The listing builds one solid part. Answer for the finished solid, in the listing's coordinates (mm). A direction names the side the tool comes from. Coordinates: 2 decimals unless noted, no trailing zeros. Order: outer loops, then holes, each group sorted by start corner. A loop starts at its lowest first (then second) coordinate and runs counter-clockwise, first axis right, second up.
from build123d import *

# Parameters (mm, degrees)
SALIENTE_EXTRUIR1_DEPTH = 8
REDONDEO3_R             = 5
REDONDEO4_R             = 5
REDONDEO5_R             = 35
REDONDEO6_R             = 10
REDONDEO7_R             = 10
VACIADO1_T              = -2
CROQUIS2_R              = 2
SALIENTE_EXTRUIR2_DEPTH = 6
CROQUIS3_R              = 5
CORTAR_EXTRUIR1_DEPTH   = 10
CROQUIS4_R              = 2
SALIENTE_EXTRUIR4_DEPTH = 6
CORTAR_EXTRUIR2_START   = 10
CORTAR_EXTRUIR2_DEPTH   = 10
CROQUIS6_R              = 2
SALIENTE_EXTRUIR5_DEPTH = 6
CROQUIS7_R              = 2.5
CORTAR_EXTRUIR3_DEPTH   = 10
CORTAR_EXTRUIR4_DEPTH   = 5
REDONDEO8_R             = 2


with BuildPart() as part:
    # Croquis1 → Saliente-Extruir1 (new body)
    with BuildSketch(Plane(origin=(0, 0, 0), x_dir=(1, 0, 0), z_dir=(0, 1, 0))):
        Polygon((-30, 0), (-30, 6.559995295), (-20.5612792, 13.970160587), (0, 5.719083833), (20.5612792, 13.970160587), (30, 6.559995295), (30, 0), (0, -34.662162162), align=None)
    extrude(amount=SALIENTE_EXTRUIR1_DEPTH)

    # Redondeo3
    redondeo3_edges = [part.edges().sort_by_distance(p)[0] for p in [
        (0, 4, 34.662162162),
    ]]
    fillet(redondeo3_edges, radius=REDONDEO3_R)

    # Redondeo4
    redondeo4_edges = [part.edges().sort_by_distance(p)[0] for p in [
        (-20.5612792, 4, -13.970160587),
        (20.5612792, 4, -13.970160587),
    ]]
    fillet(redondeo4_edges, radius=REDONDEO4_R)

    # Redondeo5
    # the kernel refuses this fillet: 35 mm, written as the material it takes off along each edge
    with BuildSketch(Plane(origin=(-30, -29.587762227, 0), x_dir=(0.6544253650435297, 0, 0.7561266042056997), z_dir=(0, 1, 0))) as redondeo5_piece_1:
        with BuildLine():
            CenterArc((11.835104891, 35), REDONDEO5_R, 241.323383223, 28.676616777)
            Line((-4.960186966, 4.293027316), (-5.296092803, 3.678887862))
            ThreePointArc((-5.296092803, 3.678887862), (-2.938191238, 1.617225035), (-0.458097756, -0.529288623))
            Line((-0.458097756, -0.529288623), (0, -0.7))
            Line((0, -0.7), (11.835104891, -0.7))
            Line((11.835104891, -0.7), (11.835104891, 0))
        make_face()
    extrude(amount=67.175524454, mode=Mode.SUBTRACT)
    with BuildSketch(Plane(origin=(30, -29.587762227, 0), x_dir=(0, 0, -1), z_dir=(0, 1, 0))) as redondeo5_piece_2:
        with BuildLine():
            CenterArc((13.956050105, 34.209623986), REDONDEO5_R, 229.12390756, 28.676616777)
            Line((-8.948837672, 7.745192839), (-9.406935427, 7.215904216))
            Line((-9.406935427, 7.215904216), (-0.458097756, -0.529288623))
            Line((-0.458097756, -0.529288623), (0, -0.7))
            ThreePointArc((0, -0.7), (3.279997647, -0.7), (6.412074199, -0.68419248))
            Line((6.412074199, -0.68419248), (6.559995295, 0))
        make_face()
    extrude(amount=67.175524454, mode=Mode.SUBTRACT)

    # Redondeo6
    redondeo6_edges = [part.edges().sort_by_distance(p)[0] for p in [
        (-30, 4, -6.559995295),
        (30, 4, -6.559995295),
    ]]
    fillet(redondeo6_edges, radius=REDONDEO6_R)

    # Redondeo7
    redondeo7_edges = [part.edges().sort_by_distance(p)[0] for p in [
        (0, 4, -5.719083833),
    ]]
    fillet(redondeo7_edges, radius=REDONDEO7_R)

    # Vaciado1
    vaciado1_openings = [part.faces().sort_by_distance(p)[0] for p in [
        (0, 8, 5.527661799),
    ]]
    offset(amount=VACIADO1_T, openings=vaciado1_openings, kind=Kind.INTERSECTION)

    # Croquis2 → Saliente-Extruir2 (add, through all)
    with BuildSketch(Plane(origin=(0, 2, 0), x_dir=(1, 0, 0), z_dir=(0, 1, 0))):
        with Locations(Location((0, -24.021871509, 0), (0, 0, 90))):
            Circle(CROQUIS2_R)
    extrude(amount=SALIENTE_EXTRUIR2_DEPTH)

    # Croquis3 → Cortar-Extruir1 (cut)
    with BuildSketch(Plane(origin=(0, 2, 0), x_dir=(1, 0, 0), z_dir=(0, 1, 0))):
        with Locations((20.168821407, 11.224565194)):
            Circle(CROQUIS3_R)
    extrude(amount=CORTAR_EXTRUIR1_DEPTH, mode=Mode.SUBTRACT)

    # Croquis4 → Saliente-Extruir4 (add, through all)
    with BuildSketch(Plane(origin=(0, 2, 0), x_dir=(1, 0, 0), z_dir=(0, 1, 0))):
        with Locations(Location((19.744313659, 8.254751535, 0), (0, 0, 90))):
            Circle(CROQUIS4_R)
    extrude(amount=SALIENTE_EXTRUIR4_DEPTH)

    # Croquis5 → Cortar-Extruir2 (cut)
    with BuildSketch(Plane(origin=(0, 2, 0), x_dir=(1, 0, 0), z_dir=(0, 1, 0)).offset(CORTAR_EXTRUIR2_START)):
        with BuildLine():
            Line((-23.915581781, 14.17421255), (-23.915581781, 8.72634885))
            ThreePointArc((-23.915581781, 8.72634885), (-23.578448406, 9.04178192), (-23.22368003, 9.33724145))
            Line((-23.22368003, 9.33724145), (-21.596854982, 10.614431735))
            ThreePointArc((-21.596854982, 10.614431735), (-20.168821407, 11.224565194), (-18.627041323, 11.038939482))
            Line((-18.627041323, 11.038939482), (-15.564418219, 9.809933346))
            Line((-15.564418219, 9.809933346), (-15.564418219, 14.17421255))
            Line((-15.564418219, 14.17421255), (-23.915581781, 14.17421255))
        make_face()
    extrude(amount=-CORTAR_EXTRUIR2_DEPTH, mode=Mode.SUBTRACT)

    # Croquis6 → Saliente-Extruir5 (add, through all)
    with BuildSketch(Plane(origin=(0, 2, 0), x_dir=(1, 0, 0), z_dir=(0, 1, 0))):
        with Locations(Location((-16.8551421, -1.672109492, 0), (0, 0, 90))):
            Circle(CROQUIS6_R)
    extrude(amount=SALIENTE_EXTRUIR5_DEPTH)

    # Croquis7 → Cortar-Extruir3 (cut)
    with BuildSketch(Plane(origin=(0, 2, 0), x_dir=(1, 0, 0), z_dir=(0, 1, 0))):
        with Locations(Location((0, -8.30592839, 0), (0, 0, 270))):
            Circle(CROQUIS7_R)
    extrude(amount=-CORTAR_EXTRUIR3_DEPTH, mode=Mode.SUBTRACT)

    # Croquis8 → Cortar-Extruir4 (cut)
    with BuildSketch(Plane(origin=(0, 2, 0), x_dir=(1, 0, 0), z_dir=(0, 1, 0))):
        with BuildLine():
            Line((2.20642721, 1.459281861), (-2.20642721, 1.459281861))
            Line((-2.20642721, 1.459281861), (-2.20642721, -5.589003848))
            ThreePointArc((-2.20642721, -5.589003848), (0, -4.80592839), (2.20642721, -5.589003848))
            Line((2.20642721, -5.589003848), (2.20642721, 1.459281861))
        make_face()
        with BuildLine():
            ThreePointArc((2.20642721, -5.589003848), (0, -4.80592839), (-2.20642721, -5.589003848))
            Line((-2.20642721, -5.589003848), (-2.20642721, -7.130479979))
            ThreePointArc((-2.20642721, -7.130479979), (0, -5.80592839), (2.20642721, -7.130479979))
            Line((2.20642721, -7.130479979), (2.20642721, -5.589003848))
        make_face()
        with BuildLine():
            Line((-2.20642721, -7.130479979), (-2.20642721, -5.589003848))
            ThreePointArc((-2.20642721, -5.589003848), (-1.504577144, -11.46603086), (3.5, -8.30592839))
            ThreePointArc((3.5, -8.30592839), (3.160102469, -6.801351246), (2.20642721, -5.589003848))
            Line((2.20642721, -5.589003848), (2.20642721, -7.130479979))
            ThreePointArc((2.20642721, -7.130479979), (2.425496653, -7.700151214), (2.5, -8.30592839))
            ThreePointArc((2.5, -8.30592839), (-0.605777176, -10.731425043), (-2.20642721, -7.130479979))
        make_face()
    extrude(amount=-CORTAR_EXTRUIR4_DEPTH, mode=Mode.SUBTRACT)

    # Redondeo8
    redondeo8_edges = [part.edges().sort_by_distance(p)[0] for p in [
        (-2.20642721, 1, 5.589003848),
        (-2.20642721, 1, -1.459281861),
        (2.20642721, 1, -1.459281861),
        (2.20642721, 1, 5.589003848),
    ]]
    fillet(redondeo8_edges, radius=REDONDEO8_R)


solid = part.part
(1) Find section A-A on y = 5. Determine the outline of the cut face in (x, z).
(2) Find section D-D on x = 11.5. Determine the outline of the cut face in (y, z) (3 decimals).
(3) Find section C-C on z = 15. Determine the outline of the cut face in (x, y), then the cut area to 3 significant figures.
(4) Find the intervals of material crossed by probe 1 along X at (y, z) = (3, 25.5); probe 2 along Y at (x, z) = (7.5, 9); probe 3 along X at (y, z) = (4.5, -3), in increasing order.
(5) The mould has two halves that part along Z. Classify faces 1 (the cylindrical face through (20.49, 1.01, -13.2)), 2 (the cylindrical face through (-25.05, 3.94, 5.25)), 3 (the flat face through (2.206, 1, 3)): pulls with the +Z half, pulls with the -Z half, needs draft (parallel to the pull), parting line crosses it, or undercut.
(6) Given pin 1 Ø2 at (x, y) = (5, 4.5) entering from -Z; pin 2 Ø1 at (y, z) = (1.5, 12.5) entering from +X; pin 3 Ø2 at (y, z) = (6, -9.5) entering from +X; pin 4 Ø12 at (x, z) = (16.5, 26) entering from -Y, each flat-ended and moving along its own axis, determine where each tip first touches the part or whether it passes through.
(7) A tool of negligible diameter and unlimited length cuts with its end or side. For faces 4 (the cylindrical face through (1.217, 4.958, 25.609)), 5 (the cylindrical face through (28.05, 4.06, -5.2)), 6 (the flat face through (-2.206, 1, 3)), from which of +Z, -Z, +X, -X, +Y, -Y can it reach the whole face along a straight path? Write none if from no direction.
(8) Find section B-B on z = 10. Determine the outline of the cut face in (x, y).
Resolved:
1. outline: (-27.28, 1.32) arc R10 ccw to (-24.46, -10.91) - (-23.92, -11.34) - (-23.92, -8.73) arc R8 cw to (-25.48, 0.45) arc R33 cw to (-20.74, 7.64) - (-2.27, 28.99) arc R3 cw to (2.27, 28.99) - (20.74, 7.64) arc R33 cw to (25.48, 0.45) arc R8 cw to (24.26, -8.36) arc R5 cw to (25.09, -10.37) arc R10 ccw to (27.28, 1.32) arc R35 ccw to (22.25, 8.95) - (3.78, 30.29) arc R5 ccw to (-3.78, 30.29) - (-22.25, 8.95) arc R35 ccw to start; circle Ø4 at (-16.86, 1.67); (-15.56, -11.96) - (-3.72, -7.21) arc R10 cw to (3.72, -7.21) - (15.2, -11.82) arc R5 cw to (15.39, -9.74) - (4.47, -5.36) arc R12 ccw to (-4.47, -5.36) - (-15.56, -9.81) - close; circle Ø4 at (0, 24.02); circle Ø4 at (19.74, -8.25)
2. outline: (0, -10.334) - (8, -10.334) - (8, -8.179) - (2, -8.179) - (2, 18.319) - (8, 18.319) - (8, 21.375) - (0, 21.375) - close
3. outline: (-17.02, 0) - (17.02, 0) - (17.02, 8) - (14.37, 8) - (14.37, 2) - (-14.37, 2) - (-14.37, 8) - (-17.02, 8) - close
3. area: 99.8 mm2
4. probe 1: x = -7.93 to -5.28, -1.35 to 1.35, 5.28 to 7.93
4. probe 2: y = 0 to 2
4. probe 3: x = -28.28 to -26.28, 26.28 to 28.28
5. face 1: pulls with the -Z half
5. face 2: pulls with the +Z half
5. face 3: undercut
6. pin 1: stops at z = -8.13
6. pin 2: stops at x = 19.61
6. pin 3: stops at x = 26.66
6. pin 4: passes through
7. face 4: +Y
7. face 5: +X, +Y, -Y
7. face 6: +Y, -Y
8. outline: (-21.35, 0) - (-3.06, 0) - (-3.06, 2) - (-18.7, 2) - (-18.7, 8) - (-21.35, 8) - close; (3.06, 0) - (21.35, 0) - (21.35, 8) - (18.7, 8) - (18.7, 2) - (3.06, 2) - close
